Geometry: final body of the model. Coordinates: model frame, mm. A direction names the side the tool comes from. Round coordinates to 2 decimals unless told otherwise and drop trailing zeros. Order: outer loops, then holes, each group sorted by start corner. A loop starts at its lowest first (then second) coordinate and runs counter-clockwise, first axis right, second up. Notation, with made-up numbers: M 20.5,70 L 52.5,70 A11 ccw 52.5,78 Z; hole C 0,-22.75 d1. An arc over 180 degrees is marked long. Return JSON: item names as keys, results as strings. Group by question number.
Q1. Access query for faces 1 (the face through (1.43, -2.75, 5.52)), 2 (the face through (-1.27, -0.97, 1.97)). Directions: +Z, -Z, +X, -X, +Y, -Y. A direction counts if a zero-diameter tool reaches every point of the face in a straight line with its end or side. Return the directions, or none.
Q2. Contact query for flat-ended pins moving along their axis: pin 1 (3 mm diameter, centred on y = 5.5, z = 1, fed in from -X); pin 2 (3 mm diameter, centred on y = -6.5, z = 5.5, fed in from +X); pin 3 (3 mm diameter, centred on x = 0, z = 6, fed in from -Y). Output: stop coordinate, or through.
Q3. Cut plane A-A on x = 0. Output: boundary loops of the cut face in (y, z), and give its area (3 significant figures).
Q4. Cut plane C-C on z = 4.5. Output: boundary loops of the cut face in (x, y).
Q5. Cut plane B-B on z = 6.5. Output: boundary loops of the cut face in (x, y), and give its area (3 significant figures).
Q6. Mould query, pull axis X, two halves, no side actions, for faces 3 (the face through (-1.355, -6.102, 6.593)), 4 (the face through (0, -4, 0)), 5 (the face through (1.3, -1.3, 4)). Classes: released by +X, released by -X, zero draft, split by the parting line, or undercut.
Q7. Ray query, probe 1 along Y at (x, z) = (-0.5, 2.75); probe 2 along X at (y, z) = (-1, 1.75); probe 3 along Z at (x, y) = (1, 11). Return the intervals inside material, ascending.
```python
from build123d import *

# Parameters (mm, degrees)
F0_R     = 17.5
F0_R_2   = 1.6
F1_DEPTH = 7
F2_R     = 3.1
F2_R_2   = 1.6
F3_DEPTH = 3
F4_SIZE2 = 6.5
F4_SIZE  = 12


with BuildPart() as f1:
    # F0 (on Top) → F1 (new body)
    with BuildSketch(Plane.XY):
        Circle(F0_R)
        Circle(F0_R_2, mode=Mode.SUBTRACT)
    extrude(amount=F1_DEPTH)

    # F2 (on face) → F3 (cut)
    with BuildSketch(Plane.XY.offset(7)):
        Circle(F2_R)
        Circle(F2_R_2, mode=Mode.SUBTRACT)
    extrude(amount=-F3_DEPTH, mode=Mode.SUBTRACT)

    # F4
    f4_edges = [f1.edges().sort_by_distance(p)[0] for p in [
        (-17.5, 0, 7),
    ]]
    f4_side = f1.faces().sort_by_distance((-17.005025, 0, 7))[0]
    chamfer(f4_edges, length=F4_SIZE, length2=F4_SIZE2, reference=f4_side)


solid = f1.part
```
Result sheet:
{
 "1": {"face 1": "+Z", "face 2": "+Z, -Z"},
 "2": {"pin 1": "stops at x = -17.02", "pin 2": "stops at x = 9.08", "pin 3": "stops at y = -10.12"},
 "3": {"outline": "M -17.5,0 L -1.6,0 L -1.6,4 L -3.1,4 L -3.1,7 L -5.5,7 L -17.5,0.5 Z; M 1.6,0 L 17.5,0 L 17.5,0.5 L 5.5,7 L 3.1,7 L 3.1,4 L 1.6,4 Z", "area": "136 mm²"},
 "4": {"outline": "C 0,0 d20.23; hole C 0,0 d6.2"},
 "5": {"outline": "C 0,0 d12.85; hole C 0,0 d6.2", "area": "99.4 mm²"},
 "6": {"face 3": "split by the parting line", "face 4": "zero draft", "face 5": "undercut"},
 "7": {"probe 1": "y = -13.34 to -1.52, 1.52 to 13.34", "probe 2": "x = -15.16 to -1.25, 1.25 to 15.16", "probe 3": "z = 0 to 4"}
}
